```python
from build123d import *

# Parameters (mm, degrees)
BASE_W_MOTOR_MOUNTS_R  = 70
BOSS_EXTRUDE1_DEPTH    = 3.175
STANDOFFS_TOP_BOTTOM_R = 1.65
CUT_EXTRUDE2_DEPTH     = 3.175


with BuildPart() as part:
    # Base w/ Motor Mounts → Boss-Extrude1 (new body)
    with BuildSketch(Plane(origin=(0, 0, 0), x_dir=(1, 0, 0), z_dir=(0, 1, 0))):
        Circle(BASE_W_MOTOR_MOUNTS_R)
    extrude(amount=BOSS_EXTRUDE1_DEPTH)

    # Standoffs (top / bottom) → Cut-Extrude2 (cut)
    with BuildSketch(Plane(origin=(0, 0, 0), x_dir=(1, 0, 0), z_dir=(0, 1, 0))):
        with Locations((25.257106536, 60.976049146)):
            Circle(STANDOFFS_TOP_BOTTOM_R)
        with Locations((60.976049146, 25.257106536)):
            Circle(STANDOFFS_TOP_BOTTOM_R)
        with Locations((60.976049146, -25.257106536)):
            Circle(STANDOFFS_TOP_BOTTOM_R)
        with Locations((25.257106536, -60.976049146)):
            Circle(STANDOFFS_TOP_BOTTOM_R)
        with Locations((-25.257106536, -60.976049146)):
            Circle(STANDOFFS_TOP_BOTTOM_R)
        with Locations((-60.976049146, -25.257106536)):
            Circle(STANDOFFS_TOP_BOTTOM_R)
        with Locations((-60.976049146, 25.257106536)):
            Circle(STANDOFFS_TOP_BOTTOM_R)
        with Locations((-25.257106536, 60.976049146)):
            Circle(STANDOFFS_TOP_BOTTOM_R)
    extrude(amount=CUT_EXTRUDE2_DEPTH, mode=Mode.SUBTRACT)


solid = part.part
```
Could you check a few things on this model? Use its own coordinates, in mm. Round coordinates to 2 decimals unless told otherwise and drop trailing zeros. Write each loop counter-clockwise with the first axis right and the second up, starting at its lowest first coordinate (ties: lowest second). Pieces come first, ordered by that corner, then holes.
(1) Thinking about a two-plate mould opening in Z: for faces 1 (the face through (-55.55, 1.565, 42.594)), 2 (the face through (-62.624, 1.565, 25.185)), 3 (the face through (-1, 0, -1)), which applies, +Z half, -Z half, draft (parallel to the pull), parting line (faces both ways), or undercut?
Findings below:
face 1: parting line
face 2: undercut
face 3: draft
(2) If I drill on probe 1 along Z at (x, y) = (-38, 2.85); probe 2 along X at (y, z) = (1.2, 6.5); probe 3 along Z at (x, y) = (-56.5, 0.9), over which ranges is the centre line in solid material (lowest first)?
Findings below:
probe 1: z = -58.79 to 58.79
probe 2: x = -69.7 to 69.7
probe 3: z = -41.32 to 41.32
(3) For pin 1 (1 mm diameter, centred on y = 2.5, z = 5, fed in from -X); pin 2 (1.5 mm diameter, centred on y = 2, z = 20.5, fed in from +X), each with a flat end and sliding along its axis, tell me the tip position at first contact or that it passes through.
Findings below:
pin 1: stops at x = -69.86
pin 2: stops at x = 67.16
(4) Suppose I cut it at C-C on x = -18. Write out the boundary of the cut face in (y, z) (3 decimals), and give its area (3 significant figures).
Findings below:
outline: (0, -67.646) - (3.175, -67.646) - (3.175, 67.646) - (0, 67.646) - close
area: 430 mm2
(5) Suppose I cut it at B-B on z = 49.5. Write out the boundary of the cut face in (x, y) (3 decimals).
Findings below:
outline: (-49.495, 0) - (49.495, 0) - (49.495, 3.175) - (-49.495, 3.175) - close
(6) Suppose I cut it at A-A on y = 1.6. State how many separate pieces and enclosed holes the cut face has, and give its area (3 significant figures).
Findings below:
separate pieces: 1
enclosed holes: 8
area: 15,300 mm2
